Model file for the job. Use its own axes, mm. Face numbers are marked on the shaded views. Round coordinates to 2 decimals unless told otherwise and drop trailing zeros. Loops run counter-clockwise (first coordinate to the right, second up) from the corner with the lowest first, then second, coordinate; pieces in that order, holes last. Notation, with made-up numbers: M 76,-9.75 L 127,-9.75 A8 ccw 127,1.25 Z; hole C -35.5,12.5 d8. An arc over 180 degrees is marked long. Answer in a Markdown table with one row per item.
from build123d import *

# Parameters (mm, degrees)
F0_R     = 63.5
F1_DEPTH = 10.16
F2_R     = 12.7
F3_DEPTH = 248.92
F5_DEPTH = 6.35


with BuildPart() as f1:
    # F0 (on Top) → F1 (new body)
    with BuildSketch(Plane.XY):
        Circle(F0_R)
    extrude(amount=F1_DEPTH)

    # F2 (on Top) → F3 (join)
    with BuildSketch(Plane.XY):
        Circle(F2_R)
    extrude(amount=F3_DEPTH)

    # F4 (on Front) → F5 (join, symmetric)
    with BuildSketch(Plane.XZ):
        Polygon((-88.9, 205.788166), (-88.9, 195.628166), (0, 195.628166), (88.9, 195.628166), (88.9, 205.788166), align=None)
        Polygon((-99.06, 195.628166), (-88.9, 195.628166), (-88.9, 205.788166), (-88.9, 214.678166), (-99.06, 214.678166), align=None)
        Polygon((88.9, 78.788166), (0, 78.788166), (0, 73.708166), (0, 68.628166), (88.9, 68.628166), align=None)
        Polygon((0, 73.708166), (0, 78.788166), (-88.9, 78.788166), (-88.9, 68.628166), (0, 68.628166), align=None)
        Polygon((88.9, 142.288166), (0, 142.288166), (0, 137.208166), (0, 132.128166), (88.9, 132.128166), align=None)
        Polygon((0, 137.208166), (0, 142.288166), (-88.9, 142.288166), (-88.9, 132.128166), (0, 132.128166), align=None)
        Polygon((88.9, 205.788166), (88.9, 195.628166), (99.06, 195.628166), (99.06, 214.678166), (88.9, 214.678166), align=None)
        Polygon((-88.9, 132.128166), (-88.9, 142.288166), (-88.9, 151.178166), (-99.06, 151.178166), (-99.06, 132.128166), align=None)
        Polygon((88.9, 151.178166), (88.9, 142.288166), (88.9, 132.128166), (99.06, 132.128166), (99.06, 151.178166), align=None)
        Polygon((-88.9, 68.628166), (-88.9, 78.788166), (-88.9, 87.678166), (-99.06, 87.678166), (-99.06, 68.628166), align=None)
        Polygon((88.9, 87.678166), (88.9, 78.788166), (88.9, 68.628166), (99.06, 68.628166), (99.06, 87.678166), align=None)
    extrude(amount=F5_DEPTH, both=True)


solid = f1.part
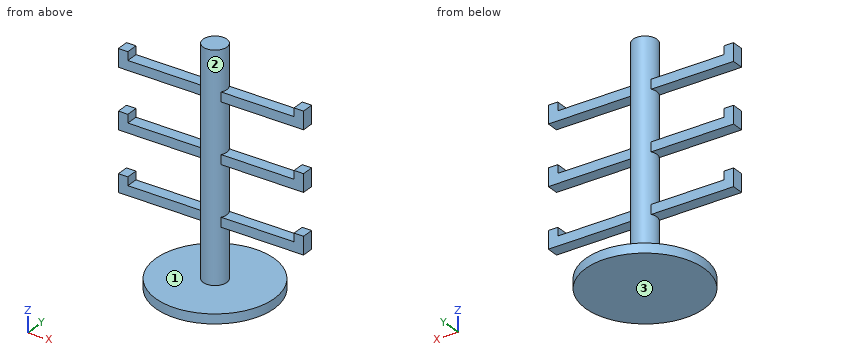
1. Wall check: probe 1 along Z at (x, y) = (62.5, -6); probe 2 along Z at (x, y) = (21, -44); probe 3 along Y at (x, z) = (-59.5, 73). Give the ranges that are in metal, low to high.
Verdict:
| item | result |
|---|---|
| probe 1 | z = 0 to 10.16, 68.63 to 78.79, 132.13 to 142.29, 195.63 to 205.79 |
| probe 2 | z = 0 to 10.16 |
| probe 3 | y = -6.35 to 6.35 |
2. Saw through at C-C (x = 0). Write the cut outline in (y, z).
Verdict:
| item | result |
|---|---|
| outline | M -63.5,0 L 63.5,0 L 63.5,10.16 L 12.7,10.16 L 12.7,248.92 L -12.7,248.92 L -12.7,10.16 L -63.5,10.16 Z |
3. Mould opens along Z. For the marked faces 1, 2 and 3 say: +Z half, -Z half, draft (parallel to the pull), parting line (faces both ways), or undercut.
Verdict:
| item | result |
|---|---|
| face 1 | undercut |
| face 2 | undercut |
| face 3 | -Z half |
4. Saw through at B-B (x = 24). Write the cut outline in (y, z), and give its area (3 significant figures).
Verdict:
| item | result |
|---|---|
| outline | M -58.79,0 L 58.79,0 L 58.79,10.16 L -58.79,10.16 Z; M -6.35,68.63 L 6.35,68.63 L 6.35,78.79 L -6.35,78.79 Z; M -6.35,132.13 L 6.35,132.13 L 6.35,142.29 L -6.35,142.29 Z; M -6.35,195.63 L 6.35,195.63 L 6.35,205.79 L -6.35,205.79 Z |
| area | 1,580 mm² |
5. Saw through at A-A (x = -68). Write the cut outline in (y, z).
Verdict:
| item | result |
|---|---|
| outline | M -6.35,68.63 L 6.35,68.63 L 6.35,78.79 L -6.35,78.79 Z; M -6.35,132.13 L 6.35,132.13 L 6.35,142.29 L -6.35,142.29 Z; M -6.35,195.63 L 6.35,195.63 L 6.35,205.79 L -6.35,205.79 Z |
6. Saw through at D-D (z = 166). Write the cut outline in (x, y).
Verdict:
| item | result |
|---|---|
| outline | C 0,0 d25.4 |
7. Pin check, flat tips, straight feed: pin 1 (8 mm diameter, centred on x = -96, y = -2.5, fed in from +Z); pin 2 (10 mm diameter, centred on x = -22.5, z = 222.5, fed in from -Y); pin 3 (10 mm diameter, centred on x = -32, y = 1, fed in from +Z); pin 4 (8 mm diameter, centred on x = 18.5, z = 77, fed in from +Y). Stop position of each tip, or through.
Verdict:
| item | result |
|---|---|
| pin 1 | stops at z = 214.68 |
| pin 2 | passes through |
| pin 3 | stops at z = 205.79 |
| pin 4 | stops at y = 6.35 |
